```python
from build123d import *

# Parameters (mm, degrees)
SKETCH2_R           = 1.5
BOSS_EXTRUDE1_DEPTH = 5
BOSS_EXTRUDE2_DEPTH = 5


with BuildPart() as part:
    # Sketch2 → Boss-Extrude1 (new body)
    with BuildSketch(Plane.XY):
        with BuildLine():
            Line((-12.5, -3.693265424), (-12.5, 25))
            Line((-12.5, 25), (12.5, 25))
            Line((12.5, 25), (12.5, -3.693265424))
            ThreePointArc((12.5, -3.693265424), (0, 0), (-12.5, -3.693265424))
        make_face()
        with Locations((-7.751243347, 8.5)):
            Circle(SKETCH2_R, mode=Mode.SUBTRACT)
        with Locations((7.751243347, 8.5)):
            Circle(SKETCH2_R, mode=Mode.SUBTRACT)
    extrude(amount=BOSS_EXTRUDE1_DEPTH)

    # Sketch3 → Boss-Extrude2 (add)
    with BuildSketch(Plane(origin=(0, 0, 0), x_dir=(-1, 0, 0), z_dir=(0, 0, -1))):
        Polygon((2.502486694, 11.5), (2.502486694, 25), (-2.502486694, 25), (-2.502486694, 11.5), (-2.502486694, 3.5), (-2.502486694, 3), (-7, 3), (-7, 0.5), (-7, 0), (7, 0), (7, 0.5), (7, 3), (2.502486694, 3), (2.502486694, 3.5), align=None)
    extrude(amount=BOSS_EXTRUDE2_DEPTH)

    # Mirror1: part across plane


with BuildPart() as part_1:
    add(part.part)
    add(part.part.mirror(Plane(origin=(-12.5, 25, 5), x_dir=(0, 0, 1), z_dir=(0, -1, 0))))

    # Mirror2: part across plane


with BuildPart() as part_2:
    add(part_1.part)
    add(part_1.part.mirror(Plane(origin=(12.5, 12.5, 0), x_dir=(0, 0, 1), z_dir=(0.7071067811865488, 0.7071067811865464, 0))))


solid = part_2.part
```
Geometry check sheet. Reference: the model listing, model coordinates, mm. A direction names the side the tool comes from. Coordinates: 2 decimals unless noted, no trailing zeros. Loops run counter-clockwise (first coordinate to the right, second up) from the corner with the lowest first, then second, coordinate; pieces in that order, holes last. Notation, with made-up numbers: (87, -27.75) -> (129, -27.75) arc R13 ccw to (129, -16.75) -> close; hole circle Ø9 at (-35.5, 38). An arc over 180 degrees is marked (long way). Put each result on its own line as item: value.
1) Release check for a two-part mould opening along Y. For faces 4 (the flat face through (-20, 12.5, 2)), 5 (the flat face through (-5, 47, -2)), 6 (the flat face through (2, 25, -5)) record: released by +Y, released by -Y, zero draft, split by the parting line, or undercut.
Result set:
face 4: released by -Y
face 5: undercut
face 6: zero draft
2) Thickness scan on line 1 (X direction, y = 41.5, z = 1.35); line 2 (X direction, y = 33, z = 4.75); line 3 (Y direction, x = 8.5, z = 4.5). Record the ranges inside material, lowest first.
Result set:
line 1: x = -12.5 to -9.25, -6.25 to 6.25, 9.25 to 12.5
line 2: x = -26.44 to -17.98, -15.02 to 15.02, 17.98 to 26.44
line 3: y = -1.63 to 7.2, 9.8 to 40.2, 42.8 to 51.63
3) Gauge pin test, flat ends, axial feed: pin 1 Ø4 at (x, y) = (-16.5, 17.25) entering from -Z; pin 2 Ø1.3 at (y, z) = (19.5, -3.5) entering from -X; pin 3 Ø2.5 at (y, z) = (6, 3) entering from -X; pin 4 Ø3.5 at (x, y) = (7.75, 8.5) entering from +Z. Record the tip position at first contact, or that the pin passes through.
Result set:
pin 1: stops at z = 0
pin 2: stops at x = -25
pin 3: stops at x = -12.5
pin 4: stops at z = 5
4) Cross-section at B-B on x = -16.5. Record the boundary of the cut face in (y, z), plus the area to 3 significant figures.
Result set:
outline: (12.5, 0) -> (15.75, 0) -> (15.75, 5) -> (12.5, 5) -> close; (18.75, 0) -> (22.5, 0) -> (22.5, -5) -> (27.5, -5) -> (27.5, 0) -> (31.25, 0) -> (31.25, 5) -> (18.75, 5) -> close; (34.25, 0) -> (37.5, 0) -> (37.5, 5) -> (34.25, 5) -> close
area: 120 mm^2
5) Cross-section at D-D on y = 2. Record the boundary of the cut face in (x, z), plus the area to 3 significant figures.
Result set:
outline: (-12.5, 0) -> (-7, 0) -> (-7, -5) -> (7, -5) -> (7, 0) -> (12.5, 0) -> (12.5, 5) -> (-12.5, 5) -> close
area: 195 mm^2
6) Tool access check on faces 1 (the flat face through (2.502, 13, -2)), 2 (the flat face through (-24, 32, -2)), 3 (the flat face through (5, 47, -2)). Record the directions out of +Z, -Z, +X, -X, +Y, -Y that give a thin tool (end or side, any length) a straight path to the whole face; none if there is none.
Result set:
face 1: -Z
face 2: -Z, -X, +Y
face 3: -Z, +X
7) Cross-section at A-A on y = 8.5. Record the boundary of the cut face in (x, z), plus the area to 3 significant figures.
Result set:
outline: (-12.5, 0) -> (-9.25, 0) -> (-9.25, 5) -> (-12.5, 5) -> close; (-6.25, 0) -> (-2.5, 0) -> (-2.5, -5) -> (2.5, -5) -> (2.5, 0) -> (6.25, 0) -> (6.25, 5) -> (-6.25, 5) -> close; (9.25, 0) -> (12.5, 0) -> (12.5, 5) -> (9.25, 5) -> close
area: 120 mm^2
8) Cross-section at C-C on z = 2.5. Count the separate pieces of the cut face and the enclosed holes in it, plus the area to 3 significant figures.
Result set:
separate pieces: 1
enclosed holes: 8
area: 1,940 mm^2
